```python
from build123d import *

# Parameters (mm, degrees)
SKETCH054_W             = 50
SKETCH054_H             = 20
PAD053_DEPTH            = 5
SKETCH055_W             = 50
SKETCH055_H             = 3
PAD054_DEPTH            = 20
SKETCH056_W             = 50
SKETCH056_H             = 10
PAD055_DEPTH            = 3
BODY042_ROLL_ANGLE      = 150.405023
BODY042_PITCH_ANGLE     = -0.370429
BODY042_PLACEMENT_ANGLE = -178.656588


with BuildPart() as part:
    # Sketch054 → Pad053 (new body)
    with BuildSketch(Plane.XY):
        with Locations((184.845276, -123.914059)):
            Rectangle(SKETCH054_W, SKETCH054_H)
    extrude(amount=PAD053_DEPTH)

    # Sketch055 (on Face6 of Pad053) → Pad054 (join)
    with BuildSketch(Plane.XY.offset(5)):
        with Locations((184.83606, -132.417099)):
            Rectangle(SKETCH055_W, SKETCH055_H)
    extrude(amount=PAD054_DEPTH)

    # Sketch056 (on Face7 of Pad054) → Pad055 (join)
    with BuildSketch(Plane(origin=(0, -113.914059, 0), x_dir=(-1, 0, 0), z_dir=(0, 1, 0))):
        with Locations((-184.841869, 9.989668)):
            Rectangle(SKETCH056_W, SKETCH056_H)
    extrude(amount=-PAD055_DEPTH)


with BuildPart() as part_1:
    # Body042 roll: moved
    add(part.part.rotate(Axis((0, 0, 0), (1, 0, 0)), BODY042_ROLL_ANGLE))


with BuildPart() as part_2:
    # Body042 pitch: moved
    add(part_1.part.rotate(Axis((0, 0, 0), (0, 1, 0)), BODY042_PITCH_ANGLE))


with BuildPart() as part_3:
    # Body042 placement: moved
    add(part_2.part.moved(Location((285.028603, 95.891543, 263.575076))).rotate(Axis((285.028603, 95.891543, 263.575076), (0, 0, 1)), BODY042_PLACEMENT_ANGLE))


solid = part_3.part
```
The model under review builds one solid part; all positions refer to its coordinate system, in mm. Round coordinates to 2 decimals unless told otherwise and drop trailing zeros. Write each loop counter-clockwise with the first axis right and the second up, starting at its lowest first coordinate (ties: lowest second). Pieces come first, ordered by that corner, then holes. Notation, with made-up numbers: (11.5, 74.5) -> (16.5, 74.5) arc R29 cw to (16.5, 107.5) -> close; hole circle Ø2 at (28, 6). An arc over 180 degrees is marked (long way). Use CSV: the item, a comma, the result in double quotes.
Q1. To check wall thickness, follow probe 1 along Z at (x, y) = (109, -14); probe 2 along Y at (x, z) = (105, 196); probe 3 along Z at (x, y) = (125, -12). State the ranges of each line that lie inside material, in increasing order. Write a range as [from, to].
Checks:
probe 1,"[179.73, 185.81], [198.92, 204.68]"
probe 2,"[-23.32, -19.29], [-3.76, -0.31]"
probe 3,"[176.77, 182.84], [199.74, 205.49]"
Q2. Consider section D-D (z = 205.5). Give the boundary of the cut face in (x, y), then the cut area to 3 significant figures.
Checks:
outline,"(77.14, -6.26) -> (77.31, -13.65) -> (127.29, -11.91) -> (127.13, -5.27) -> close"
area,"351 mm²"
Q3. For pin 1 Ø3 at (x, z) = (94, 184) entering from -Y; pin 2 Ø8 at (x, z) = (99, 201.5) entering from +Y; pin 3 Ø12 at (x, y) = (113, -19.5) entering from -Z, all flat-tipped, find the tip position at first contact; note any pin that passes through.
Checks:
pin 1,"y = -17.57"
pin 2,"y = -1.28"
pin 3,"z = 178.99"
Q4. Consider section A-A (y = -15). Give the boundary of the cut face in (x, z), then the cut area to 3 significant figures.
Checks:
outline,"(77.19, 180.38) -> (127.22, 182.13) -> (127.26, 188.2) -> (77.23, 186.46) -> close; (77.3, 198.98) -> (127.31, 197.99) -> (127.35, 203.74) -> (77.34, 204.73) -> close"
area,"591 mm²"
Q5. Consider section C-C (z = 182.5). Give the boundary of the cut face in (x, y).
Checks:
outline,"(77.15, -12.75) -> (77.23, -16.2) -> (127.23, -15.21) -> (127.15, -11.76) -> close"
